For this review, take the finished solid that the model builds, in its own axes (mm). A direction names the side the tool comes from. Give positions to 0.01 mm unless a question says otherwise; leave off trailing zeros. Order: outer loops, then holes, each group sorted by start corner. A loop starts at its lowest first (then second) coordinate and runs counter-clockwise, first axis right, second up. Notation, with made-up numbers: M -24.5,-20.75 L 30.5,-20.75 A18 cw 30.5,-13.75 Z; hole C 52,-24.5 d5. An arc over 180 degrees is marked long. Answer as CSV lines item,"result". Start each with the question number.
1. We need section A-A, the plane x = 27.4. Give the boundary of the cut face in (y, z), and give its area (3 significant figures).
2. For line 1 along Y through (x, z) = (27.4, 4.45); line 2 along Y through (x, z) = (27.4, 1.55); line 3 along X through (y, z) = (90.4, 2.2), list the stretches that pass through material, from the lowest coordinate up.
3. Mouldability with a two-part tool opening along X and no side actions: class faces 4 (the flat face through (31.4, -5, 3)), 5 (the cylindrical face through (-1.521, 18.14, 4.797)), 6 (the flat face through (0, 2, 4)) as pulls with the +X half, pulls with the -X half, needs draft (parallel to the pull), parting line crosses it, or undercut.
4. We need section C-C, the plane x = 47. Give the boundary of the cut face in (y, z).
5. Clearance check with flat-ended pins moving along their axes: P1, Ø3, axis at x = 49.5, z = 3, coming from the +Y side; P2, Ø4, axis at x = 27.4, y = 90.4, coming from the +Z side; P3, Ø12, axis at x = 25, y = 11.5, coming from the +Z side; P4, Ø10, axis at x = 19.5, y = 77, coming from the +Z side. State where each tip first meets the part, or that it passes through.
6. Machinability: for faces 1 (the flat face through (54.8, 81, 4)), 2 (the cylindrical face through (-1.521, 76.94, 4.797)), 3 (the flat face through (3, 42, 1)), which of the approach directions +Z, -Z, +X, -X, +Y, -Y give a long, thin tool a straight path to every point of the face, cutting with its end or side? Answer none if there is none.
7. We need section B-B, the plane y = 73. Give the boundary of the cut face in (x, z).
8. We need section D-D, the plane z = 4.8. State how many separate pieces and enclosed holes the cut face has, and give its area (3 significant figures).
Autodesk Fusion 360 part; units mm, degrees
sketch "Sketch4" plane through (0, 0, 0) normal (0, 0, 1) x (1, 0, 0)
  line L0 (0, 0) -> (54.8, 0)
  line L1 (54.8, 0) -> (54.8, 82.8)
  line L2 (54.8, 82.8) -> (0, 82.8)
  line L3 (0, 82.8) -> (0, 0)
  line L4 (57.8, -3) -> (57.8, 85.8)
  line L5 (-3, 85.8) -> (-3, -3)
  line L6 (0, 41.4) -> (54.8, 41.4) construction
  line L7 (27.4, 0) -> (27.4, 1.8094) construction
  line L8 (27.4, 1.8094) -> (27.4, 82.8) construction
  line L9 (23.4, 85.8) -> (23.4, 90.4)
  line L10 (31.4, 90.4) -> (31.4, 85.8)
  line L11 (23.4, -3) -> (23.4, -7.6)
  line L12 (31.4, -7.6) -> (31.4, -3)
  arc A0 (31.4, 90.4) -> (23.4, 90.4) centre (27.4, 90.4) ccw
  arc A1 (23.4, -7.6) -> (31.4, -7.6) centre (27.4, -7.6) ccw
  line L13 (-3, -3) -> (23.4, -3)
  line L14 (31.4, -3) -> (57.8, -3)
  line L15 (57.8, 85.8) -> (31.4, 85.8)
  line L16 (23.4, 85.8) -> (-3, 85.8)
  line L17 (3, 3) -> (51.8, 3)
  line L18 (51.8, 3) -> (51.8, 79.8)
  line L19 (51.8, 79.8) -> (3, 79.8)
  line L20 (3, 79.8) -> (3, 3)
  point P0 (27.4, 90.4)
  point P1 (27.4, -7.6)
  dimension "d22" = 54.8
  dimension "d23" = 82.8
  dimension "d25" = 8
  dimension "d26" = 49
  dimension "d27" = 49
  dimension "d30" = -3
extrude "Extrude5" add sketch "Sketch4" along normal blind 2 contours L0 L1 L2 L3
extrude "Extrude6" add sketch "Sketch4" along normal blind 6 contours L4 L5 L9 L10 L11 L12 A0 A1 L13 L14 L15 L16
sketch "Sketch5" plane through (0, 0, 6) normal (0, 0, 1) x (-1, 0, 0)
  line L0 (0, 0) -> (0, -82.8)
  line L1 (0, -82.8) -> (-54.8, -82.8)
  line L2 (-54.8, -82.8) -> (-54.8, 0)
  line L3 (-54.8, 0) -> (0, 0)
  arc A0 (-31.4, -90.4) -> (-23.4, -90.4) centre (-27.4, -90.4) ccw
  line L4 (-23.4, -90.4) -> (-23.4, -85.8)
  line L5 (-23.4, -85.8) -> (3, -85.8)
  line L6 (3, -85.8) -> (3, 3)
  line L7 (3, 3) -> (-23.4, 3)
  line L8 (-23.4, 3) -> (-23.4, 7.6)
  arc A1 (-23.4, 7.6) -> (-31.4, 7.6) centre (-27.4, 7.6) ccw
  line L9 (-31.4, 7.6) -> (-31.4, 3)
  line L10 (-31.4, 3) -> (-57.8, 3)
  line L11 (-57.8, 3) -> (-57.8, -85.8)
  line L12 (-57.8, -85.8) -> (-31.4, -85.8)
  line L13 (-31.4, -85.8) -> (-31.4, -90.4)
  circle A2 centre (-27.4, -90.4) radius 3
  circle A3 centre (-27.4, 7.6) radius 3
  dimension "d35" = 6
extrude "Extrude7" cut sketch "Sketch5" against normal blind 3 contours A2 | A3
sketch "Sketch6" plane through (0, 0, 3) normal (0, 0, 1) x (-1, 0, 0)
  circle A0 centre (-27.4, -90.4) radius 3
  circle A1 centre (-27.4, -90.4) radius 1.6
  circle A2 centre (-27.4, 7.6) radius 1.6
  dimension "d38" = 3.2
  dimension "d39" = 3.2
extrude "Extrude8" cut sketch "Sketch6" against normal blind 4 contours A1 | A2
sketch "Sketch7" plane through (0, 0, 6) normal (0, 0, 1) x (-1, 0, 0)
  circle A0 centre (-27.4, -90.4) radius 3
  circle A1 centre (-27.4, 7.6) radius 3
  line L0 (0, 0) -> (0, -82.8)
  line L1 (0, -82.8) -> (-54.8, -82.8)
  line L2 (-54.8, -82.8) -> (-54.8, 0)
  line L3 (-54.8, 0) -> (0, 0)
  arc A2 (-31.4, -90.4) -> (-23.4, -90.4) centre (-27.4, -90.4) ccw
  line L4 (-23.4, -90.4) -> (-23.4, -85.8)
  line L5 (-23.4, -85.8) -> (3, -85.8)
  line L6 (3, -85.8) -> (3, 3)
  line L7 (3, 3) -> (-23.4, 3)
  line L8 (-23.4, 3) -> (-23.4, 7.6)
  arc A3 (-23.4, 7.6) -> (-31.4, 7.6) centre (-27.4, 7.6) ccw
  line L9 (-31.4, 7.6) -> (-31.4, 3)
  line L10 (-31.4, 3) -> (-57.8, 3)
  line L11 (-57.8, 3) -> (-57.8, -85.8)
  line L12 (-57.8, -85.8) -> (-31.4, -85.8)
  line L13 (-31.4, -85.8) -> (-31.4, -90.4)
  line L14 (4.5, -17) -> (-1.5, -17)
  line L15 (-1.5, -17) -> (-1.5, -7)
  line L16 (-1.5, -7) -> (4.5, -7)
  line L17 (4.5, -7) -> (4.5, -17)
  line L18 (4.5, -17) -> (-1.5, -7) construction
  line L19 (-1.5, -17) -> (4.5, -7) construction
  line L20 (3, -41.4) -> (-57.8, -41.4) construction
  line L21 (-27.4, 0) -> (-27.4, -82.8) construction
  line L22 (-1.5, -75.8) -> (4.5, -75.8)
  line L23 (4.5, -75.8) -> (4.5, -65.8)
  line L24 (-1.5, -65.8) -> (-1.5, -75.8)
  line L25 (4.5, -65.8) -> (-1.5, -65.8)
  line L26 (0, 0) -> (-9, 0)
  line L27 (-9, 0) -> (-9, 3)
  line L28 (-9, 3) -> (0, 3)
  line L29 (0, 3) -> (0, 0)
  line L30 (-54.8, 0) -> (-45.8, 0)
  line L31 (-45.8, 3) -> (-54.8, 3)
  line L32 (-54.8, 3) -> (-54.8, 0)
  line L33 (-45.8, 0) -> (-45.8, 3)
  line L34 (-29.9523, 2.9079) -> (-24.9523, 2.9079)
  line L35 (-24.9523, 2.9079) -> (-24.9523, -0.0921)
  line L36 (-24.9523, -0.0921) -> (-29.9523, -0.0921)
  line L37 (-29.9523, -0.0921) -> (-29.9523, 2.9079)
  line L38 (-29.9523, 2.9079) -> (-24.9523, -0.0921) construction
  line L39 (-24.9523, 2.9079) -> (-29.9523, -0.0921) construction
  line L40 (-24.9523, -82.7079) -> (-29.9523, -82.7079)
  line L41 (-24.9523, -85.7079) -> (-24.9523, -82.7079)
  line L42 (-29.9523, -85.7079) -> (-24.9523, -85.7079)
  line L43 (-29.9523, -82.7079) -> (-29.9523, -85.7079)
  line L44 (0, -82.8) -> (-9, -82.8)
  line L45 (-9, -82.8) -> (-9, -85.8)
  line L46 (-9, -85.8) -> (0, -85.8)
  line L47 (0, -85.8) -> (0, -82.8)
  line L48 (-45.8, -82.8) -> (-45.8, -85.8)
  line L49 (-45.8, -85.8) -> (-54.8, -85.8)
  line L50 (-54.8, -85.8) -> (-54.8, -82.8)
  line L51 (-54.8, -82.8) -> (-45.8, -82.8)
  line L52 (-59.3, -65.8) -> (-53.3, -65.8)
  line L53 (-53.3, -65.8) -> (-53.3, -75.8)
  line L54 (-53.3, -75.8) -> (-59.3, -75.8)
  line L55 (-59.3, -75.8) -> (-59.3, -65.8)
  line L56 (-53.3, -17) -> (-53.3, -7)
  line L57 (-53.3, -7) -> (-59.3, -7)
  line L58 (-59.3, -7) -> (-59.3, -17)
  line L59 (-59.3, -17) -> (-53.3, -17)
  point P0 (1.5, -12)
  point P1 (-27.4523, 1.4079)
  dimension "d42" = 10
  dimension "d43" = 12
  dimension "d44" = 9
  dimension "d45" = 5
  dimension "d46" = 3
extrude "Extrude9" cut sketch "Sketch7" against normal blind 4 contours L3 L7 L26 L27 L28 L29 | L0 L6 L14 L16 | L0 L14 L15 L16 | L6 L14 L16 L17 | L3 L34 L35 L37 | L0 L6 L22 L25 | L0 L22 L24 L25 | L6 L22 L23 L25 | L3 L10 L30 L31 L32 L33 | L1 L5 L44 L45 L46 L47 | L2 L56 L57 L59 | L2 L11 L57 L59 | L1 L41 L42 L43 | L11 L57 L58 L59 | L2 L52 L53 L54 | L2 L11 L52 L54 | L1 L12 L48 L49 L50 L51 | L11 L52 L54 L55
fillet "Empalme4" radius 4 20 edges at (56.3, 17, 6) (56.3, 7, 6) (56.3, -3, 6) (45.8, -1.5, 6) (29.9523, -1.454, 6) (24.9523, -1.454, 6) (9, -1.5, 6) (-1.5, -3, 6) (-1.5, 7, 6) (-1.5, 17, 6) (56.3, 65.8, 6) (56.3, 75.8, 6) (56.3, 85.8, 6) (45.8, 84.3, 6) (29.9523, 84.254, 6) (24.9523, 84.254, 6) (-1.5, 75.8, 6) (-1.5, 65.8, 6) (-1.5, 85.8, 6) (9, 84.3, 6)
Result set:
1,outline,"M -11.6,0 L -9.2,0 L -9.2,3 L -10.6,3 L -10.6,6 L -11.6,6 Z; M -6,0 L 3,0 L 3,2 L -2.91,2 L -2.91,6 L -4.6,6 L -4.6,3 L -6,3 Z; M 79.8,0 L 88.8,0 L 88.8,3 L 87.4,3 L 87.4,6 L 85.71,6 L 85.71,2 L 79.8,2 Z; M 92,0 L 94.4,0 L 94.4,6 L 93.4,6 L 93.4,3 L 92,3 Z"
1,area,"72.7 mm2"
2,line 1,"-11.6 to -10.6, -4.6 to -2.91, 85.71 to 87.4, 93.4 to 94.4"
2,line 2,"-11.6 to -9.2, -6 to 3, 79.8 to 88.8, 92 to 94.4"
2,line 3,"23.4 to 25.8, 29 to 31.4"
3,face 4,"pulls with the +X half"
3,face 5,"needs draft"
3,face 6,"undercut"
4,outline,"M -3,0 L 3,0 L 3,2 L -3,2 Z; M 79.8,0 L 85.8,0 L 85.8,2 L 79.8,2 Z"
5,P1,"y = 85.8"
5,P2,"z = 3"
5,P3,"through"
5,P4,"z = 2"
6,face 1,"+Z, +Y, -Y"
6,face 2,"+Z, +X, -X"
6,face 3,"+Z, -Z"
7,outline,"M -3,0 L 3,0 L 3,2 L -3,2 Z; M 51.8,0 L 57.8,0 L 57.8,2 L 51.8,2 Z"
8,separate pieces,"8"
8,enclosed holes,"2"
8,area,"604 mm2"
